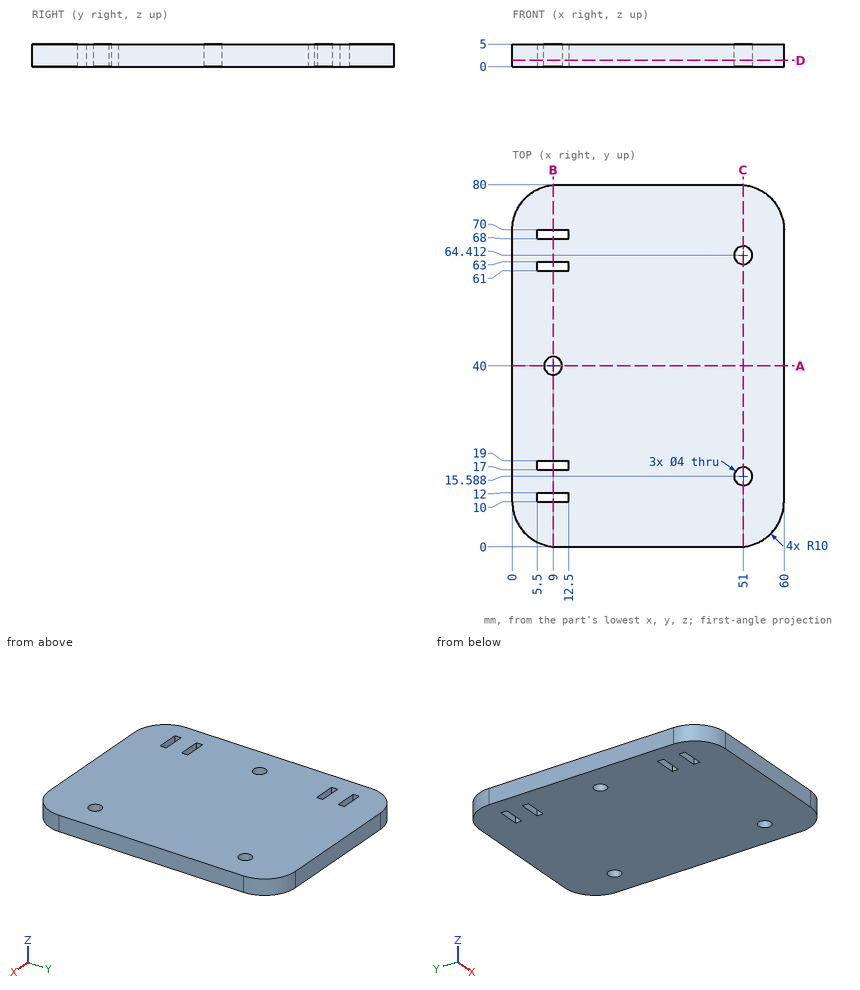
Study the drawing (mm; zero at the part's minimum x, y, z) and answer. Coordinates: 2 decimals unless noted, no trailing zeros. Write each loop counter-clockwise with the first axis right and the second up, starting at its lowest first coordinate (ties: lowest second). Pieces come first, ordered by that corner, then holes.
Q1. Find the intervals of material crossed by line 1 (Y direction, x = 51, z = 3.9); line 2 (Y direction, x = 9, z = 3.5); line 3 (Y direction, x = 8, z = 3.6), in increasing order.
Q2. A cutting plane is placed at B-B, the plane x = 9. Give the vertices of the cut face in (y, z).
Q3. A cutting plane is placed at C-C, the plane x = 51. Give the vertices of the cut face in (y, z).
Q4. Each of these flat-tipped pins is pushed along its axis until it touches: pin 1 Ø3 at (x, z) = (52, 0.5) entering from +Y; pin 2 Ø1 at (y, z) = (69, 3.5) entering from -X; pin 3 Ø1.5 at (x, z) = (8, 3.5) entering from -Y; pin 4 Ø2 at (y, z) = (8, 3.5) entering from +X. Where does it stop, or does it pass through?
Q5. A cutting plane is placed at A-A, the plane y = 40. Give the vertices of the cut face in (x, z), then the cut area to 3 significant figures.
Q6. A cutting plane is placed at D-D, the plane z = 1.4. Give the vertices of the cut face in (x, y), then the cut area to 3 significant figures.
Findings below:
1. line 1: y = 0.05 to 13.59, 17.59 to 62.41, 66.41 to 79.95
1. line 2: y = 0.05 to 10, 12 to 17, 19 to 38, 42 to 61, 63 to 68, 70 to 79.95
1. line 3: y = 0.2 to 10, 12 to 17, 19 to 38.27, 41.73 to 61, 63 to 68, 70 to 79.8
2. outline: (0.05, 0) - (10, 0) - (10, 5) - (0.05, 5) - close; (12, 0) - (17, 0) - (17, 5) - (12, 5) - close; (19, 0) - (38, 0) - (38, 5) - (19, 5) - close; (42, 0) - (61, 0) - (61, 5) - (42, 5) - close; (63, 0) - (68, 0) - (68, 5) - (63, 5) - close; (70, 0) - (79.95, 0) - (79.95, 5) - (70, 5) - close
3. outline: (0.05, 0) - (13.59, 0) - (13.59, 5) - (0.05, 5) - close; (17.59, 0) - (62.41, 0) - (62.41, 5) - (17.59, 5) - close; (66.41, 0) - (79.95, 0) - (79.95, 5) - (66.41, 5) - close
4. pin 1: stops at y = 79.99
4. pin 2: stops at x = 0
4. pin 3: stops at y = 0.08
4. pin 4: stops at x = 59.95
5. outline: (0, 0) - (7, 0) - (7, 5) - (0, 5) - close; (11, 0) - (60, 0) - (60, 5) - (11, 5) - close
5. area: 280 mm2
6. outline: (0, 10) arc R10 ccw to (10, 0) - (50, 0) arc R10 ccw to (60, 10) - (60, 70) arc R10 ccw to (50, 80) - (10, 80) arc R10 ccw to (0, 70) - close; hole (5.5, 10) - (12.5, 10) - (12.5, 12) - (5.5, 12) - close; hole (5.5, 17) - (12.5, 17) - (12.5, 19) - (5.5, 19) - close; hole (5.5, 61) - (12.5, 61) - (12.5, 63) - (5.5, 63) - close; hole (5.5, 68) - (12.5, 68) - (12.5, 70) - (5.5, 70) - close; hole circle Ø4 at (9, 40); hole circle Ø4 at (51, 15.59); hole circle Ø4 at (51, 64.41)
6. area: 4,620 mm2
